Could you check a few things on this model? Use its own coordinates, in mm. Face numbers are marked on the shaded views. A direction names the side the tool comes from. Coordinates: 2 decimals unless noted, no trailing zeros. Loops run counter-clockwise (first coordinate to the right, second up) from the corner with the lowest first, then second, coordinate; pieces in that order, holes last. Notation, with made-up numbers: (68, -20) - (101, -20) arc R25 ccw to (101, 15) - close; hole circle Ø6 at (71.25, 8.5). An arc over 180 degrees is marked (long way). Put each result on its own line as item: value. Start each with the question number.
```python
from build123d import *

# Parameters (mm, degrees)
PAD008_DEPTH         = 13
POCKET012_DEPTH      = 20.501
POCKET012_DEPTH_BACK = 20.501
SKETCH037_W          = 20
SKETCH037_H          = 63.5
PAD012_DEPTH         = 20
POCKET020_DEPTH      = 20.501
POCKET020_DEPTH_BACK = 20.501
THICKNESS_T          = 1
SKETCH028_W          = 20
SKETCH028_H          = 7
SKETCH028_W_2        = 28.5
SKETCH028_H_2        = 10
POCKET021_DEPTH      = 5
SKETCH029_W          = 9
SKETCH029_H          = 3
SKETCH029_W_2        = 9.0000000001
SKETCH029_H_2        = 4
PAD013_DEPTH         = 12
SKETCH030_R          = 1.75
POCKET022_DEPTH      = 59.0010001
POCKET023_DEPTH      = 2
SKETCH041_W          = 1
SKETCH041_H          = 38
PAD016_DEPTH         = 15


with BuildPart() as part:
    # Sketch020 → Pad008 (new body)
    with BuildSketch(Plane.XY):
        with BuildLine():
            Line((-13.5, 0), (-13.5, -10))
            Line((-13.5, -10), (-20.5, -10))
            Line((-20.5, -10), (-20.5, 4.5))
            ThreePointArc((-15.25, 9.75), (-18.9623106012, 8.2123106012), (-20.5, 4.5))
            ThreePointArc((-15.25, 9.7500000001), (-11.5376893988, 11.2876893988), (-10, 15))
            Line((-10, 15), (10, 15))
            ThreePointArc((10, 15), (11.5376893988, 11.2876893988), (15.25, 9.75))
            ThreePointArc((20.5, 4.5), (18.9623106012, 8.2123106012), (15.25, 9.75))
            Line((20.5, -10), (20.5, 4.5))
            Line((13.5, -10), (20.5, -10))
            Line((13.5, 0), (13.5, -10))
            Line((13.5, 0), (13.5, 3))
            ThreePointArc((13.5, 3), (12.767766953, 4.767766953), (11, 5.5))
            Line((-11, 5.5), (11, 5.5))
            ThreePointArc((-11, 5.5), (-12.767766953, 4.767766953), (-13.5, 3))
            Line((-13.5, 0), (-13.5, 3))
        make_face()
    extrude(amount=PAD008_DEPTH)

    # Sketch021 → Pocket012 (cut, two sides)
    with BuildSketch(Plane.YZ) as pocket012_sk:
        Polygon((-10, 4), (-5, 4), (10, 19), (-10, 19), align=None)
    extrude(amount=-POCKET012_DEPTH, mode=Mode.SUBTRACT)
    extrude(pocket012_sk.sketch, amount=POCKET012_DEPTH_BACK, mode=Mode.SUBTRACT)

    # Sketch037 → Pad012 (join)
    with BuildSketch(Plane.XY):
        with Locations((0, 46.75)):
            Rectangle(SKETCH037_W, SKETCH037_H)
    extrude(amount=PAD012_DEPTH)

    # Sketch038 → Pocket020 (cut, two sides)
    with BuildSketch(Plane.YZ) as pocket020_sk:
        with BuildLine():
            Line((15, 33), (15, 13))
            add(Edge.make_bspline(
                [(15, 13), (23.5, 13), (23.5, 15), (32, 15)],
                knots=[0, 0, 0, 0, 1, 1, 1, 1], degree=3))
            Line((32, 15), (61, 15))
            ThreePointArc((61, 15), (62.767766953, 15.732233047), (63.5, 17.5))
            Line((63.5, 17.5), (63.5, 33))
            Line((63.5, 33), (15, 33))
        make_face()
        with BuildLine():
            add(Edge.make_bspline(
                [(15, 0), (23.5, 0), (23.5, 2), (32, 2)],
                knots=[0, 0, 0, 0, 1, 1, 1, 1], degree=3))
            Line((32, 2), (71, 2))
            ThreePointArc((71, 2), (76.3033008589, 4.1966991411), (78.5, 9.5))
            Line((78.5, 9.5), (78.5, 33))
            Line((78.5, 33), (98.5, 33))
            Line((98.5, 33), (98.5, 0))
            Line((98.5, 0), (15, 0))
        make_face()
    extrude(amount=-POCKET020_DEPTH, mode=Mode.SUBTRACT)
    extrude(pocket020_sk.sketch, amount=POCKET020_DEPTH_BACK, mode=Mode.SUBTRACT)

    # Thickness
    thickness_openings = [part.faces().sort_by_distance(p)[0] for p in [
        (0, 71, 20),
    ]]
    offset(amount=THICKNESS_T, openings=thickness_openings, kind=Kind.INTERSECTION)

    # Sketch028 (on DatumPlane) → Pocket021 (cut)
    with BuildSketch(Plane.XY.offset(2.5)):
        with Locations((0, 3.5)):
            Rectangle(SKETCH028_W, SKETCH028_H)
        with Locations((0, -5)):
            Rectangle(SKETCH028_W_2, SKETCH028_H_2)
    extrude(amount=-POCKET021_DEPTH, mode=Mode.SUBTRACT)

    # Sketch029 (on DatumPlane) → Pad013 (join)
    with BuildSketch(Plane.XY.offset(1.5)):
        with Locations((14.5, 22)):
            Rectangle(SKETCH029_W, SKETCH029_H)
        with Locations((-14.5, 22)):
            Rectangle(SKETCH029_W, SKETCH029_H)
        with Locations((14.5, 58.5)):
            Rectangle(SKETCH029_W_2, SKETCH029_H_2)
    extrude(amount=PAD013_DEPTH)

    # Sketch030 (on DatumPlane) → Pocket022 (cut, through all)
    with BuildSketch(Plane(origin=(0, 20.5, 0), x_dir=(-1, 0, 0), z_dir=(0, 1, 0))):
        with Locations((-15.5, 8)):
            Circle(SKETCH030_R)
        with Locations((15, 8)):
            Circle(SKETCH030_R)
    extrude(amount=POCKET022_DEPTH, mode=Mode.SUBTRACT)

    # Sketch035 (on DatumPlane) → Pocket023 (cut)
    with BuildSketch(Plane(origin=(0, 56.5, 0), x_dir=(-1, 0, 0), z_dir=(0, 1, 0))):
        Polygon((-12.6854174377, 6.375), (-12.6854174377, 9.625), (-15.5, 11.25), (-18.3145825623, 9.625), (-18.3145825623, 6.375), (-15.5, 4.75), align=None)
    extrude(amount=POCKET023_DEPTH, mode=Mode.SUBTRACT)

    # Sketch041 (on DatumPlane) → Pad016 (join)
    with BuildSketch(Plane.XY.offset(1)):
        with Locations((-4, 51)):
            Rectangle(SKETCH041_W, SKETCH041_H)
        with Locations((4, 51)):
            Rectangle(SKETCH041_W, SKETCH041_H)
    extrude(amount=PAD016_DEPTH)


with BuildPart() as part_1:
    # Body003 placement: moved
    add(part.part.moved(Location((4, -20.5, -32))))


solid = part_1.part
```
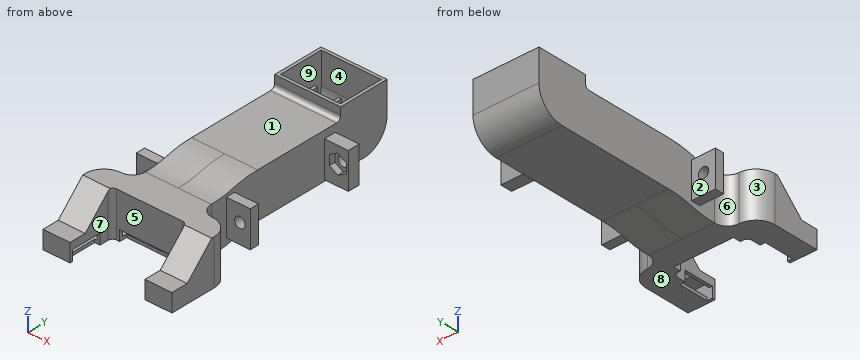
(1) If we mould it in two halves opening along X, with no side actions, what happens to the marked faces 6, 7, 8 and 9? For each: pulls with the +X half, pulls with the -X half, needs draft (parallel to the pull), parting line crosses it, or undercut.
(2) For pin 1 Ø0.5 at (x, z) = (0, -24) entering from +Y; pin 2 Ø2 at (x, z) = (-10, -28) entering from +Y; pin 3 Ø4 at (x, z) = (19.5, -24) entering from +Y, each with a flat end and sliding along its axis, tell me the tip position at first contact or that it passes through.
(3) I need wall thicknesses on L1, parallel to X at y = 2.1, z = -24; L2, parallel to X at y = 38.85, z = -24; L3, parallel to X at y = 16, z = -20.25. Which ranges of each line are inside material? Lowest first, please. Write a range as [from, to].
(4) I want a section at B-B on z = -24. Count the separate pieces of the cut face and the enclosed holes in it, and give its area (3 significant figures).
(5) I want a section at A-A on y = -23.5. List the corners of the cut face in (x, z) for me.
(6) Which directions (+Z, -Z, +X, -X, +Y, -Y) give clear straight access to the entire face, cutting with the end or side of a thin tool? Please do the marked faces 1, 2, 3, 4 and 5.
Answer sheet:
1. face 6: pulls with the -X half
1. face 7: undercut
1. face 8: needs draft
1. face 9: undercut
2. pin 1: stops at y = 58.91
2. pin 2: stops at y = 3
2. pin 3: stops at y = 40
3. L1: x = [-15, -12.75], [-9.25, -6], [14, 17.75], [21.25, 23]
3. L2: x = [-7, -6], [-0.5, 0.5], [7.5, 8.5], [14, 17.75], [21.25, 23]
3. L3: x = [-7, -6], [-0.5, 0.5], [7.5, 8.5], [14, 15]
4. separate pieces: 6
4. enclosed holes: 1
4. area: 372 mm^2
5. outline: (-17.5, -33) - (-10.25, -33) - (-10.25, -32) - (-16.5, -32) - (-16.5, -26) - (-9.5, -26) - (-9.5, -29.5) - (-8.5, -29.5) - (-8.5, -24.59) - (-17.5, -24.59) - close; (16.5, -29.5) - (17.5, -29.5) - (17.5, -26) - (24.5, -26) - (24.5, -32) - (18.25, -32) - (18.25, -33) - (25.5, -33) - (25.5, -24.59) - (16.5, -24.59) - close
6. face 1: +Z, +X, -X, -Y
6. face 2: +Z, -Z, -X, +Y
6. face 3: +Z, -Z, -X
6. face 4: +Z
6. face 5: +Z, -Z, -Y
